```python
from build123d import *

# Parameters (mm, degrees)
F0_W     = 236
F0_H     = 256
F0_R     = 4.5
F0_R_2   = 5
F0_R_3   = 55
F1_DEPTH = 8
F2_SIZE  = 0.5


with BuildPart() as f1:
    # F0 (on Top) → F1 (new body)
    with BuildSketch(Plane.XY):
        Rectangle(F0_W, F0_H)
        with Locations((-98, -119)):
            Circle(F0_R, mode=Mode.SUBTRACT)
        with Locations((-45.961941, -45.961941)):
            Circle(F0_R, mode=Mode.SUBTRACT)
        with Locations((0, -119)):
            Circle(F0_R_2, mode=Mode.SUBTRACT)
        with Locations((98, -119)):
            Circle(F0_R, mode=Mode.SUBTRACT)
        with Locations((45.961941, -45.961941)):
            Circle(F0_R, mode=Mode.SUBTRACT)
        with Locations((-45.961941, 45.961941)):
            Circle(F0_R, mode=Mode.SUBTRACT)
        with Locations((-98, 119)):
            Circle(F0_R, mode=Mode.SUBTRACT)
        Circle(F0_R_3, mode=Mode.SUBTRACT)
        with Locations((45.961941, 45.961941)):
            Circle(F0_R, mode=Mode.SUBTRACT)
        with Locations((0, 119)):
            Circle(F0_R_2, mode=Mode.SUBTRACT)
        with Locations((98, 119)):
            Circle(F0_R, mode=Mode.SUBTRACT)
    extrude(amount=F1_DEPTH)

    # F2
    f2_edges = [f1.edges().sort_by_distance(p)[0] for p in [
        (-93.5, -119, 4),
        (-102.5, -119, 0),
        (-102.5, -119, 8),
        (-41.461941, -45.961941, 4),
        (-50.461941, -45.961941, 0),
        (-50.461941, -45.961941, 8),
        (55, 0, 4),
        (-55, 0, 0),
        (-55, 0, 8),
        (-41.461941, 45.961941, 4),
        (-50.461941, 45.961941, 0),
        (-50.461941, 45.961941, 8),
        (50.461941, -45.961941, 4),
        (41.461941, -45.961941, 0),
        (41.461941, -45.961941, 8),
        (102.5, -119, 4),
        (93.5, -119, 0),
        (93.5, -119, 8),
        (-93.5, 119, 4),
        (-102.5, 119, 0),
        (-102.5, 119, 8),
        (50.461941, 45.961941, 4),
        (41.461941, 45.961941, 0),
        (41.461941, 45.961941, 8),
        (102.5, 119, 4),
        (93.5, 119, 0),
        (93.5, 119, 8),
        (5, 119, 4),
        (-5, 119, 0),
        (-5, 119, 8),
        (5, -119, 4),
        (-5, -119, 0),
        (-5, -119, 8),
    ]]
    chamfer(f2_edges, length=F2_SIZE)


solid = f1.part
```
Part model, mm, in its own coordinate system. Round coordinates to 2 decimals unless told otherwise and drop trailing zeros. Loops run counter-clockwise (first coordinate to the right, second up) from the corner with the lowest first, then second, coordinate; pieces in that order, holes last.
1. Two-plate mould, pull along X, no slides. Class faces 1 (the face through (-2, 128, 4)), 2 (the face through (118, -2, 4)), 3 (the face through (-102.496, -118.802, 3.951)): pulls with the +X half, pulls with the -X half, needs draft (parallel to the pull), parting line crosses it, or undercut.
Solutions:
face 1: needs draft
face 2: pulls with the +X half
face 3: undercut
2. Drill centre lines: line 1 along Y through (x, z) = (-98, 5.5); line 2 along Y through (x, z) = (0, 3); line 3 along Y through (x, z) = (42, 0.5). Where is each one in solid material? Low to high.
Solutions:
line 1: y = -128 to -123.5, -114.5 to 114.5, 123.5 to 128
line 2: y = -128 to -124, -114 to -55, 55 to 114, 124 to 128
line 3: y = -128 to -48.1, -43.83 to -35.51, 35.51 to 43.83, 48.1 to 128
3. Slice it at A-A (x = 0). Give the cut face in (y, z).
Solutions:
outline: (-128, 0) - (-124.5, 0) - (-124, 0.5) - (-124, 7.5) - (-124.5, 8) - (-128, 8) - close; (-114, 0.5) - (-113.5, 0) - (-55.5, 0) - (-55, 0.5) - (-55, 7.5) - (-55.5, 8) - (-113.5, 8) - (-114, 7.5) - close; (55, 0.5) - (55.5, 0) - (113.5, 0) - (114, 0.5) - (114, 7.5) - (113.5, 8) - (55.5, 8) - (55, 7.5) - close; (124, 0.5) - (124.5, 0) - (128, 0) - (128, 8) - (124.5, 8) - (124, 7.5) - close
4. Slice it at C-C (x = 98). Give the cut face in (y, z), and give its area (3 significant figures).
Solutions:
outline: (-128, 0) - (-124, 0) - (-123.5, 0.5) - (-123.5, 7.5) - (-124, 8) - (-128, 8) - close; (-114.5, 0.5) - (-114, 0) - (114, 0) - (114.5, 0.5) - (114.5, 7.5) - (114, 8) - (-114, 8) - (-114.5, 7.5) - close; (123.5, 0.5) - (124, 0) - (128, 0) - (128, 8) - (124, 8) - (123.5, 7.5) - close
area: 1,900 mm2
5. Slice it at B-B (y = -119). Give the cut face in (x, z).
Solutions:
outline: (-118, 0) - (-103, 0) - (-102.5, 0.5) - (-102.5, 7.5) - (-103, 8) - (-118, 8) - close; (-93.5, 0.5) - (-93, 0) - (-5.5, 0) - (-5, 0.5) - (-5, 7.5) - (-5.5, 8) - (-93, 8) - (-93.5, 7.5) - close; (5, 0.5) - (5.5, 0) - (93, 0) - (93.5, 0.5) - (93.5, 7.5) - (93, 8) - (5.5, 8) - (5, 7.5) - close; (102.5, 0.5) - (103, 0) - (118, 0) - (118, 8) - (103, 8) - (102.5, 7.5) - close
6. Slice it at D-D (z = 2). Count the separate pieces of the cut face and the enclosed holes in it, and give its area (3 significant figures).
Solutions:
separate pieces: 1
enclosed holes: 11
area: 50,200 mm2
7. Flat gauge pin, fed straight in: pin 1 (7 mm diameter, centred on x = -98, y = -119, fed in from -Z). Where does the tip first touch, or does it go through?
Solutions:
pin 1: passes through
